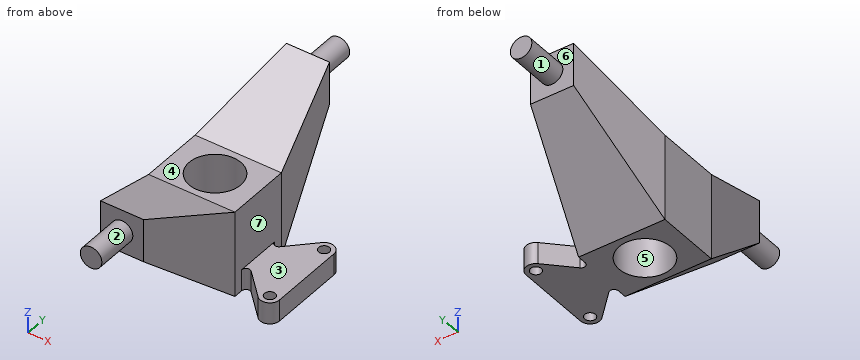
```python
from build123d import *

# Parameters (mm, degrees)
ESQUISSE1_W        = 40
ESQUISSE1_H        = 30
ESQUISSE1_R        = 12
BOSS_EXTRU_1_DEPTH = 40
ESQUISSE3_R        = 5
BOSS_EXTRU_2_DEPTH = 20
ESQUISSE4_R        = 2.5
BOSS_EXTRU_3_DEPTH = 10
CONG_1_R           = 2
CONG_2_R           = 2


with BuildPart() as part:
    # Esquisse1 → Boss.-Extru.1 (new body)
    with BuildSketch(Plane.XY):
        Rectangle(ESQUISSE1_W, ESQUISSE1_H)
        Circle(ESQUISSE1_R, mode=Mode.SUBTRACT)
    extrude(amount=-BOSS_EXTRU_1_DEPTH)

    # Esquisse2 → section 0 of lissage1
    with BuildSketch(Plane(origin=(0, 60, 0), x_dir=(1, 0, 0), z_dir=(0, 1, 0)), mode=Mode.PRIVATE) as lissage1_s0:
        with BuildLine():
            Line((10, 0), (-10, 0))
            Line((-10, 0), (-10, -20))
            Line((-10, -20), (10, -20))
            Line((10, -20), (10, 0))
        make_face()
    # loft up to a face of the part (lissage1)
    loft([lissage1_s0.sketch, part.faces().sort_by_distance((0, 15, -20))[0]])

    # Esquisse3 → Boss.-Extru.2 (add)
    with BuildSketch(Plane(origin=(0, 60, 0), x_dir=(1, 0, 0), z_dir=(0, 1, 0))):
        with Locations(Location((0, -10, 0), (0, 0, 270))):
            Circle(ESQUISSE3_R)
    extrude(amount=BOSS_EXTRU_2_DEPTH)

    # Symétrie7: part across plane


with BuildPart() as part_1:
    add(part.part)
    add(part.part.mirror(Plane.ZX))

    # Esquisse4 → Boss.-Extru.3 (add)
    with BuildSketch(Plane(origin=(0, 0, -40), x_dir=(-1, 0, 0), z_dir=(0, 0, -1))):
        with BuildLine():
            Line((-20, 5.863961031), (-34.818019485, 20.681980515))
            ThreePointArc((-34.818019485, 20.681980515), (-39.722075446, 21.657457896), (-42.5, 17.5))
            Line((-42.5, 17.5), (-42.5, -17.5))
            ThreePointArc((-42.5, -17.5), (-39.722075446, -21.657457896), (-34.818019485, -20.681980515))
            Line((-34.818019485, -20.681980515), (-20, -5.863961031))
            Line((-20, -5.863961031), (-20, 5.863961031))
        make_face()
        with Locations((-38, 17.5)):
            Circle(ESQUISSE4_R, mode=Mode.SUBTRACT)
        with Locations((-38, -17.5)):
            Circle(ESQUISSE4_R, mode=Mode.SUBTRACT)
    extrude(amount=-BOSS_EXTRU_3_DEPTH)

    # Congé1
    cong_1_edges = [part_1.edges().sort_by_distance(p)[0] for p in [
        (20, 5.863961031, -35),
    ]]
    fillet(cong_1_edges, radius=CONG_1_R)

    # Congé2
    cong_2_edges = [part_1.edges().sort_by_distance(p)[0] for p in [
        (20, -5.863961031, -35),
    ]]
    fillet(cong_2_edges, radius=CONG_2_R)


solid = part_1.part
```
CAD build for the part. Positions are in the model's coordinates, mm. Face numbers are marked on the shaded views. A direction names the side the tool comes from. Round coordinates to 2 decimals unless told otherwise and drop trailing zeros. Write each loop counter-clockwise with the first axis right and the second up, starting at its lowest first coordinate (ties: lowest second). Pieces come first, ordered by that corner, then holes. Notation, with made-up numbers: (45, -5.5) - (78, -5.5) arc R3 ccw to (78, -1.5) - close; hole circle Ø1 at (54, 53.5). An arc over 180 degrees is marked (long way). Return JSON: item names as keys, results as strings. Group by question number.
Item 1: Band-saw the part on B-B on y = 0. List the corners of the cut face in (x, z), plus the area to 3 significant figures.
Item 2: Flat gauge pins, fed straight in: pin 1 Ø6 at (y, z) = (-36, -24) entering from -X; pin 2 Ø5 at (y, z) = (-18.5, -9.5) entering from +X; pin 3 Ø8 at (y, z) = (-11.5, 1.5) entering from +X; pin 4 Ø3 at (x, y) = (38, 17.5) entering from -Z. Where does each tip first touch, or does it go through?
Item 3: Probe probe 1 along Y at (x, z) = (38, -36); probe 2 along X at (y, z) = (-10, -31); probe 3 along Z at (x, y) = (35.5, -1). List the from-to ranges inside material, lowest first.
Item 4: Mould opens along Y. For the marked faces 4, 5, 6 and 7 say: +Y half, -Y half, draft (parallel to the pull), parting line (faces both ways), or undercut.
Item 5: 3-axis set-ups, long thin cutter, end or side, ignore diameter. For the marked faces 1, 2 and 3: which of +Z, -Z, +X, -X, +Y, -Y reach the whole face in a straight line?
Item 6: Band-saw the part on A-A on x = 38. List the corners of the cut face in (y, z), plus the area to 3 significant figures.
Resolved:
{
 "1": {"outline": "(-20, -40) - (-12, -40) - (-12, 0) - (-20, 0) - close; (12, -40) - (42.5, -40) - (42.5, -30) - (20, -30) - (20, 0) - (12, 0) - close", "area": "865 mm²"},
 "2": {"pin 1": "stops at x = -16", "pin 2": "stops at x = 19.78", "pin 3": "stops at x = 20", "pin 4": "passes through"},
 "3": {"probe 1": "y = -22 to -20, -15 to 15, 20 to 22", "probe 2": "x = -20 to -6.63, 6.63 to 20.12, 24.14 to 42.5", "probe 3": "z = -40 to -30"},
 "4": {"face 4": "undercut", "face 5": "undercut", "face 6": "+Y half", "face 7": "draft"},
 "5": {"face 1": "+Y", "face 2": "-Y", "face 3": "+Z, +X, +Y, -Y"},
 "6": {"outline": "(-22, -40) - (-20, -40) - (-20, -30) - (-22, -30) - close; (-15, -40) - (15, -40) - (15, -30) - (-15, -30) - close; (20, -40) - (22, -40) - (22, -30) - (20, -30) - close", "area": "340 mm²"}
}
